```python
from build123d import *

# Parameters (mm, degrees)
SKETCH2_R           = 1.8
CUT_EXTRUDE1_DEPTH  = 11
CUT_EXTRUDE2_DEPTH  = 5
SKETCH4_OUTSIDE_W   = 143.43
SKETCH4_OUTSIDE_H   = 143.43
SKETCH4_OUTSIDE_R   = 42.925
CUT_EXTRUDE3_DEPTH  = 17.3
SKETCH6_R           = 40.075
CUT_EXTRUDE5_DEPTH  = 81.915326113
CHAMFER1_SIZE       = 0.5
CUT_EXTRUDE6_DEPTH  = 3.5
CUT_EXTRUDE7_DEPTH  = 3
SKETCH9_R           = 1.75
CUT_EXTRUDE9_DEPTH  = 5
CUT_EXTRUDE10_DEPTH = 0.5


with BuildPart() as part:
    # Sketch1 → Revolve1 (revolve)
    with BuildSketch(Plane(origin=(0, 0, 0), x_dir=(1, 0, 0), z_dir=(0, 1, 0))):
        Polygon((35, 0), (35, -22.3), (55, -22.3), (55, -17.3), (49, -17.3), (49, 0), align=None)
    revolve(axis=Axis((0, 0, 94.21875), (0, 0, -1)))

    # Sketch2 → Cut-Extrude1 (cut)
    with BuildSketch(Plane.XY.offset(22.3)):
        with Locations((0, 50)):
            Circle(SKETCH2_R)
        with Locations((43.301270189, 25)):
            Circle(SKETCH2_R)
        with Locations((43.301270189, -25)):
            Circle(SKETCH2_R)
        with Locations((0, -50)):
            Circle(SKETCH2_R)
        with Locations((-43.301270189, -25)):
            Circle(SKETCH2_R)
        with Locations((-43.301270189, 25)):
            Circle(SKETCH2_R)
    extrude(amount=-CUT_EXTRUDE1_DEPTH, mode=Mode.SUBTRACT)

    # Sketch3 → Cut-Extrude2 (cut)
    with BuildSketch(Plane.XY):
        with BuildLine():
            Line((2.5, 48.936182932), (2.5, 34.910600109))
            ThreePointArc((2.5, 34.910600109), (0, 35), (-2.5, 34.910600109))
            Line((-2.5, 34.910600109), (-2.5, 48.936182932))
            ThreePointArc((-2.5, 48.936182932), (0, 49), (2.5, 48.936182932))
        make_face()
    extrude(amount=CUT_EXTRUDE2_DEPTH, mode=Mode.SUBTRACT)

    # Sketch4 outside → Cut-Extrude3 (cut)
    with BuildSketch(Plane(origin=(0, 0, 0), x_dir=(-1, 0, 0), z_dir=(0, 0, -1))):
        Rectangle(SKETCH4_OUTSIDE_W, SKETCH4_OUTSIDE_H)
        Circle(SKETCH4_OUTSIDE_R, mode=Mode.SUBTRACT)
    extrude(amount=-CUT_EXTRUDE3_DEPTH, mode=Mode.SUBTRACT)

    # Sketch6 → Cut-Extrude5 (cut, through all)
    with BuildSketch(Plane.XY):
        with Locations(Location((0, 0, 0), (0, 0, 93.576606812))):
            Circle(SKETCH6_R)
    extrude(amount=CUT_EXTRUDE5_DEPTH, mode=Mode.SUBTRACT)

    # Chamfer1
    chamfer1_edges = [part.edges().sort_by_distance(p)[0] for p in [
        (2.5, 41.424540979, 0),
        (0, -40.075, 0),
        (-2.5, 41.424540979, 0),
        (29.455416522, -31.223934129, 0),
    ]]
    chamfer(chamfer1_edges, length=CHAMFER1_SIZE)

    # Sketch7 → Cut-Extrude6 (cut)
    with BuildSketch(Plane.XY.offset(22.3)):
        Polygon((31.359931864, -20.316995311), (34.134931864, -25.123436302), (58.38364317, -11.123436302), (55.60864317, -6.316995311), align=None)
    extrude(amount=-CUT_EXTRUDE6_DEPTH, mode=Mode.SUBTRACT)

    # Sketch8 → Cut-Extrude7 (cut)
    with BuildSketch(Plane.XY.offset(22.3)):
        Polygon((-29.034798369, -30.160254038), (-30.636945366, -32.935254038), (-33.84123936, -32.935254038), (-35.443386357, -30.160254038), (-33.84123936, -27.385254038), (-30.636945366, -27.385254038), align=None)
        Polygon((-43.84123936, -10.064745962), (-45.443386357, -12.839745962), (-43.84123936, -15.614745962), (-40.636945366, -15.614745962), (-39.034798369, -12.839745962), (-40.636945366, -10.064745962), align=None)
    extrude(amount=-CUT_EXTRUDE7_DEPTH, mode=Mode.SUBTRACT)

    # Sketch9 → Cut-Extrude9 (cut)
    with BuildSketch(Plane.XY.offset(22.3)):
        with Locations((-42.239092363, -12.839745962)):
            Circle(SKETCH9_R)
        with Locations(Location((-32.239092363, -30.160254038, 0), (0, 0, 358.221796194))):
            Circle(SKETCH9_R)
    extrude(amount=-CUT_EXTRUDE9_DEPTH, mode=Mode.SUBTRACT)

    # Sketch10 → Cut-Extrude10 (cut)
    with BuildSketch(Plane.XY.offset(22.3)):
        Polygon((30.997431864, -19.689126893), (34.497431864, -25.75130472), (59.162085788, -11.511160138), (55.662085788, -5.448982311), align=None)
    extrude(amount=-CUT_EXTRUDE10_DEPTH, mode=Mode.SUBTRACT)


solid = part.part
```
The listing builds one solid part. Answer for the finished solid, in the listing's coordinates (mm). A direction names the side the tool comes from. Round coordinates to 2 decimals unless told otherwise and drop trailing zeros. Loops run counter-clockwise (first coordinate to the right, second up) from the corner with the lowest first, then second, coordinate; pieces in that order, holes last.
1) For faces 1 (the face through (-11.923, 53.692, 19.765)), 2 (the face through (44, -20, 21.8)), determine the directions among +Z, -Z, +X, -X, +Y, -Y from which every point of the face is accessible in a straight line to the end or side of a thin tool.
Outcome:
face 1: +Z, -Z
face 2: +Z
2) Consider line 1 (Y direction, x = 0, z = 18.95) (3 decimals); line 2 (X direction, y = 0, z = 12) (3 decimals); line 3 (Y direction, x = -34, z = 20.5). Determine where each line is inside the solid, lowest interval first.
Outcome:
line 1: y = -55 to -51.8, -48.2 to -40.075, 40.075 to 48.2, 51.8 to 55
line 2: x = -42.925 to -40.075, 40.075 to 42.925
line 3: y = -43.23 to -32.66, -27.66 to -21.21, 21.21 to 43.23
3) A cutting plane is placed at B-B on y = -50. Determine the outline of the cut face in (x, z).
Outcome:
outline: (-22.91, 17.3) - (-1.8, 17.3) - (-1.8, 22.3) - (-22.91, 22.3) - close; (1.8, 17.3) - (22.91, 17.3) - (22.91, 22.3) - (1.8, 22.3) - close
4) Given P1, Ø1, axis at y = -34, z = 3, coming from the +X side; P2, Ø2, axis at y = 13, z = 11, coming from the -X side; P3, Ø4, axis at y = 15, z = 18, coming from the +X side, each flat-ended and moving along its own axis, determine where each tip first touches the part or whether it passes through.
Outcome:
P1: stops at x = 26.84
P2: stops at x = -41.21
P3: stops at x = 53.44
5) A cutting plane is placed at A-A on x = 0. Determine the outline of the cut face in (y, z) (3 decimals), plus the area to 3 significant figures.
Outcome:
outline: (-55, 17.3) - (-51.8, 17.3) - (-51.8, 22.3) - (-55, 22.3) - close; (-48.2, 17.3) - (-42.925, 17.3) - (-42.925, 0.5) - (-42.425, 0) - (-40.575, 0) - (-40.075, 0.5) - (-40.075, 22.3) - (-48.2, 22.3) - close; (40.075, 5) - (42.925, 5) - (42.925, 17.3) - (48.2, 17.3) - (48.2, 22.3) - (40.075, 22.3) - close; (51.8, 17.3) - (55, 17.3) - (55, 22.3) - (51.8, 22.3) - close
area: 197 mm2
6) A cutting plane is placed at D-D on y = 25. Give the number of separate pieces and of enclosed holes in the cut face, plus the area to 3 significant figures.
Outcome:
separate pieces: 4
enclosed holes: 0
area: 264 mm2
7) A cutting plane is placed at C-C on z = 12.5. Determine the outline of the cut face in (x, y) (3 decimals), plus the area to 3 significant figures.
Outcome:
outline: circle Ø85.85 at (0, 0); hole circle Ø80.15 at (0, 0)
area: 743 mm2
8) For a pull along Y with two mould halves and no side action, classify faces 3 (the face through (9.305, -41.904, 8.782)), 4 (the face through (41, 0, 0)), 5 (the face through (-39.825, -11.472, 20.821)) as released by +Y, released by -Y, zero draft, split by the parting line, or undercut.
Outcome:
face 3: split by the parting line
face 4: zero draft
face 5: undercut
